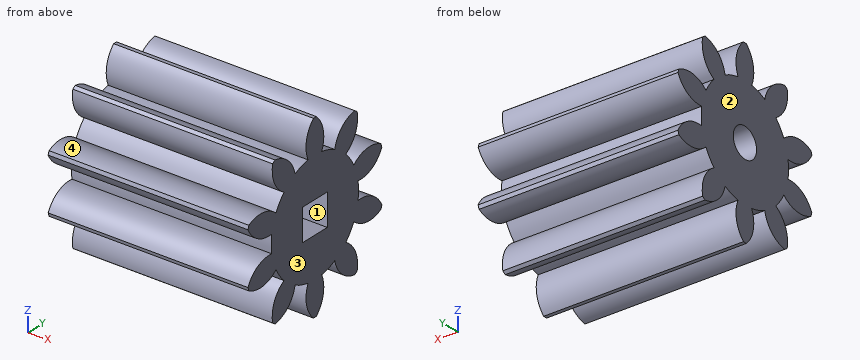
from build123d import *

# Parameters (mm, degrees)
BASPROSKE_W        = 20
BASPROSKE_H        = 9
TOOTHCUT_DEPTH     = 24.706539182
TEETHCUTS_COUNT    = 10
TEETHCUTS_ANGLE    = 324
BORSKE_R           = 1.5
BORE_DEPTH         = 50.0000508
SKETCH1_W          = 3.2
SKETCH1_H          = 3.2
CUT_EXTRUDE1_DEPTH = 10


with BuildPart() as part:
    # BasProSke → Base-Revolve (revolve)
    with BuildSketch(Plane(origin=(0, 0, 0), x_dir=(1, 0, 0), z_dir=(0, 1, 0)), mode=Mode.PRIVATE) as base_revolve_sk:
        with Locations((10, 4.5)):
            Rectangle(BASPROSKE_W, BASPROSKE_H)
    revolve(base_revolve_sk.sketch.rotate(Axis((-10, 0, 0), (1, 0, 0)), 180), axis=Axis((-10, 0, 0), (1, 0, 0)))

    # TooCutSke → ToothCut (cut, through all)
    with BuildSketch(Plane(origin=(0, 0, 0), x_dir=(0, 0, -1), z_dir=(1, 0, 0))):
        with BuildLine():
            ThreePointArc((0.883878355, 5.554109745), (0, 5.624), (-0.883878355, 5.554109745))
            ThreePointArc((-0.883878355, 5.554109745), (-1.258245767, 7.379188248), (-2.637816971, 8.631324741))
            ThreePointArc((-2.637816971, 8.631324741), (0, 9.0254), (2.637816971, 8.631324741))
            ThreePointArc((2.637816971, 8.631324741), (1.258245767, 7.379188248), (0.883878355, 5.554109745))
        make_face()
    toothcut = extrude(amount=TOOTHCUT_DEPTH, mode=Mode.SUBTRACT)

    # TeethCuts: ToothCut ×10 about axis
    teethcuts_axis = Axis((-10, 0, 0), (1, 0, 0))
    for i in range(1, TEETHCUTS_COUNT):
        add(toothcut.rotate(teethcuts_axis, i * TEETHCUTS_ANGLE / (TEETHCUTS_COUNT - 1)), mode=Mode.SUBTRACT)

    # BorSke → Bore (cut, symmetric)
    with BuildSketch(Plane(origin=(0, 0, 0), x_dir=(0, 0, -1), z_dir=(1, 0, 0))):
        with Locations(Location((0, 0, 0), (0, 0, 180))):
            Circle(BORSKE_R)
    extrude(amount=BORE_DEPTH, both=True, mode=Mode.SUBTRACT)

    # Sketch1 → Cut-Extrude1 (cut)
    with BuildSketch(Plane(origin=(20, 0, 0), x_dir=(0, 0, -1), z_dir=(1, 0, 0))):
        Rectangle(SKETCH1_W, SKETCH1_H)
    extrude(amount=-CUT_EXTRUDE1_DEPTH, mode=Mode.SUBTRACT)


solid = part.part
Verification items for the finished model (mm, model axes). Face numbers are marked on the shaded views. A direction names the side the tool comes from. Round coordinates to 2 decimals unless told otherwise and drop trailing zeros. Order: outer loops, then holes, each group sorted by start corner. A loop starts at its lowest first (then second) coordinate and runs counter-clockwise, first axis right, second up. Notation, with made-up numbers: (84.25, 70) -> (100.25, 70) arc R23 cw to (100.25, 102) -> close; hole circle Ø11 at (60.5, 36). An arc over 180 degrees is marked (long way). Put each result on its own line as item: value.
1) Mould release check, pull along Y, two halves, no side actions. Record for the marked faces 3 and 4: +Y half, -Y half, draft (parallel to the pull), parting line (faces both ways), or undercut.
Final values:
face 3: draft
face 4: undercut
2) Section check A-A (z = 0). Record the cut outline in (x, y), then the cut area to 3 significant figures.
Final values:
outline: (0, -5.62) -> (20, -5.62) -> (20, -1.6) -> (10, -1.6) -> (10, -1.5) -> (0, -1.5) -> close; (0, 1.5) -> (10, 1.5) -> (10, 1.6) -> (20, 1.6) -> (20, 5.62) -> (0, 5.62) -> close
area: 163 mm^2
3) Material ranges on line 1 (Y direction, x = 7.25, z = 0); line 2 (Z direction, x = 17, y = 4.75); line 3 (Y direction, x = 12, z = -0.5), recorded low to high.
Final values:
line 1: y = -5.62 to -1.5, 1.5 to 5.62
line 2: z = -7.32 to -4.61, -3.01 to 3.01, 4.61 to 7.32
line 3: y = -5.6 to -1.6, 1.6 to 5.6
4) Depth check by flat-ended pin: pin 1 (6 mm diameter, centred on x = 13.5, y = 5, fed in from +Z); pin 2 (1 mm diameter, centred on x = 4.5, z = 2, fed in from +Y); pin 3 (6 mm diameter, centred on x = 11, z = 6.5, fed in from -Y). Enter the tip coordinate at first touch or a pass-through.
Final values:
pin 1: stops at z = 7.39
pin 2: stops at y = 8.57
pin 3: stops at y = -5.5
5) Section check C-C (y = -3.5). Record the cut outline in (x, z).
Final values:
outline: (0, -6.65) -> (20, -6.65) -> (20, 6.65) -> (0, 6.65) -> close
6) Section check B-B (y = 4.25). Record the cut outline in (x, z), then the cut area to 3 significant figures.
Final values:
outline: (0, -7.14) -> (20, -7.14) -> (20, -4.16) -> (0, -4.16) -> close; (0, -3.68) -> (20, -3.68) -> (20, 3.68) -> (0, 3.68) -> close; (0, 4.16) -> (20, 4.16) -> (20, 7.14) -> (0, 7.14) -> close
area: 267 mm^2
7) Set-up check for the marked faces 1 and 2: record each of +Z, -Z, +X, -X, +Y, -Y from which the full face is reachable in a straight line by a thin tool's end or side.
Final values:
face 1: +X
face 2: +Z, -Z, -X, +Y, -Y
